Verification items for the finished model (mm, model axes). Coordinates: 2 decimals unless noted, no trailing zeros. Order: outer loops, then holes, each group sorted by start corner. A loop starts at its lowest first (then second) coordinate and runs counter-clockwise, first axis right, second up. Notation, with made-up numbers: (-34.75, 66.5) -> (9.25, 66.5) arc R30 ccw to (9.25, 94.5) -> close; hole circle Ø1 at (4.25, 38.25). An arc over 180 degrees is marked (long way). Answer as CSV lines item,"result".
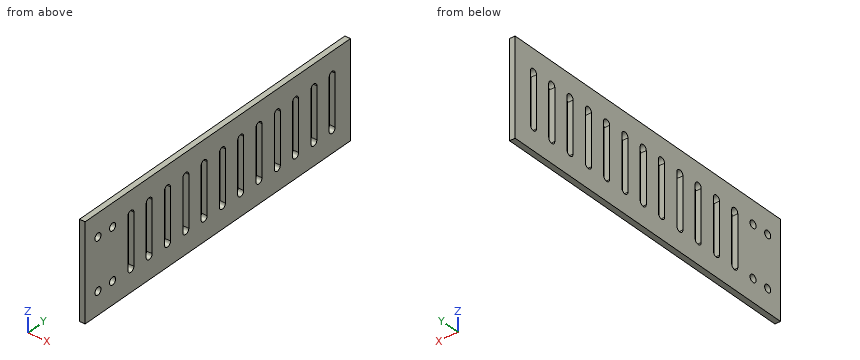
Autodesk Inventor part; units mm, degrees
ref_plane "YZ Plane" through (0, 0, 0) normal (1, 0, 0) x (0, 1, 0)
ref_plane "XZ Plane" through (0, 0, 0) normal (0, 1, 0) x (-1, 0, 0)
ref_plane "XY Plane" through (0, 0, 0) normal (0, 0, 1) x (1, 0, 0)
sketch "Sketch1" plane through (0, 0, 0) normal (1, 0, 0) x (0, 1, 0)
  circle A0 centre (0, -22.5) radius 1.65
  circle A1 centre (-8, 0) radius 1.65
  circle A2 centre (-8, -22.5) radius 1.65
  line L0 (0, 0) -> (-15, 0)
  line L1 (-15, 0) -> (-15, -22.5)
  line L2 (0, -22.5) -> (0, 0)
  line L3 (-15, -22.5) -> (-15, -32.5)
  line L4 (-15, -32.5) -> (0, -32.5)
  line L5 (0, -32.5) -> (0, -22.5)
  line L6 (0, 0) -> (-15, 0)
  line L7 (-15, 0) -> (-15, 10)
  line L8 (-15, 10) -> (0, 10)
  line L9 (0, 10) -> (0, 0)
  line L10 (0, 10) -> (130, 10)
  line L11 (130, 10) -> (130, -32.5)
  line L12 (130, -32.5) -> (0, -32.5)
  line L13 (0, -32.5) -> (0, 10)
  line L14 (10, 0) -> (10, -22.5) construction
  line L15 (8.35, 0) -> (8.35, -22.5)
  line L16 (11.65, -22.5) -> (11.65, 0)
  arc A3 (11.65, 0) -> (8.35, 0) centre (10, 0) ccw
  arc A4 (8.35, -22.5) -> (11.65, -22.5) centre (10, -22.5) ccw
  line L17 (18.35, 0) -> (18.35, -22.5)
  line L18 (20, 0) -> (20, -22.5) construction
  line L19 (21.65, -22.5) -> (21.65, 0)
  arc A5 (21.65, 0) -> (18.35, 0) centre (20, 0) ccw
  arc A6 (18.35, -22.5) -> (21.65, -22.5) centre (20, -22.5) ccw
  line L20 (28.35, 0) -> (28.35, -22.5)
  line L21 (30, 0) -> (30, -22.5) construction
  line L22 (31.65, -22.5) -> (31.65, 0)
  arc A7 (31.65, 0) -> (28.35, 0) centre (30, 0) ccw
  arc A8 (28.35, -22.5) -> (31.65, -22.5) centre (30, -22.5) ccw
  line L23 (38.35, 0) -> (38.35, -22.5)
  line L24 (40, 0) -> (40, -22.5) construction
  line L25 (41.65, -22.5) -> (41.65, 0)
  arc A9 (41.65, 0) -> (38.35, 0) centre (40, 0) ccw
  arc A10 (38.35, -22.5) -> (41.65, -22.5) centre (40, -22.5) ccw
  line L26 (48.35, 0) -> (48.35, -22.5)
  line L27 (50, 0) -> (50, -22.5) construction
  line L28 (51.65, -22.5) -> (51.65, 0)
  arc A11 (51.65, 0) -> (48.35, 0) centre (50, 0) ccw
  arc A12 (48.35, -22.5) -> (51.65, -22.5) centre (50, -22.5) ccw
  line L29 (58.35, 0) -> (58.35, -22.5)
  line L30 (60, 0) -> (60, -22.5) construction
  line L31 (61.65, -22.5) -> (61.65, 0)
  arc A13 (61.65, 0) -> (58.35, 0) centre (60, 0) ccw
  arc A14 (58.35, -22.5) -> (61.65, -22.5) centre (60, -22.5) ccw
  line L32 (68.35, 0) -> (68.35, -22.5)
  line L33 (70, 0) -> (70, -22.5) construction
  line L34 (71.65, -22.5) -> (71.65, 0)
  arc A15 (71.65, 0) -> (68.35, 0) centre (70, 0) ccw
  arc A16 (68.35, -22.5) -> (71.65, -22.5) centre (70, -22.5) ccw
  line L35 (78.35, 0) -> (78.35, -22.5)
  line L36 (80, 0) -> (80, -22.5) construction
  line L37 (81.65, -22.5) -> (81.65, 0)
  arc A17 (81.65, 0) -> (78.35, 0) centre (80, 0) ccw
  arc A18 (78.35, -22.5) -> (81.65, -22.5) centre (80, -22.5) ccw
  line L38 (88.35, 0) -> (88.35, -22.5)
  line L39 (90, 0) -> (90, -22.5) construction
  line L40 (91.65, -22.5) -> (91.65, 0)
  arc A19 (91.65, 0) -> (88.35, 0) centre (90, 0) ccw
  arc A20 (88.35, -22.5) -> (91.65, -22.5) centre (90, -22.5) ccw
  line L41 (98.35, 0) -> (98.35, -22.5)
  line L42 (100, 0) -> (100, -22.5) construction
  line L43 (101.65, -22.5) -> (101.65, 0)
  arc A21 (101.65, 0) -> (98.35, 0) centre (100, 0) ccw
  arc A22 (98.35, -22.5) -> (101.65, -22.5) centre (100, -22.5) ccw
  line L44 (108.35, 0) -> (108.35, -22.5)
  line L45 (110, 0) -> (110, -22.5) construction
  line L46 (111.65, -22.5) -> (111.65, 0)
  arc A23 (111.65, 0) -> (108.35, 0) centre (110, 0) ccw
  arc A24 (108.35, -22.5) -> (111.65, -22.5) centre (110, -22.5) ccw
  line L47 (118.35, 0) -> (118.35, -22.5)
  line L48 (120, 0) -> (120, -22.5) construction
  line L49 (121.65, -22.5) -> (121.65, 0)
  arc A25 (121.65, 0) -> (118.35, 0) centre (120, 0) ccw
  arc A26 (118.35, -22.5) -> (121.65, -22.5) centre (120, -22.5) ccw
  circle A27 centre (0, 0) radius 1.65
  point P0 (10, -11.25)
  point P1 (20, -11.25)
  point P2 (30, -11.25)
  point P3 (40, -11.25)
  point P4 (50, -11.25)
  point P5 (60, -11.25)
  point P6 (70, -11.25)
  point P7 (80, -11.25)
  point P8 (90, -11.25)
  point P9 (100, -11.25)
  point P10 (110, -11.25)
  point P11 (120, -11.25)
  dimension "d1" = 3.3
  dimension "d3" = 3.3
  dimension "d5" = 3.3
  dimension "d6" = 10
  dimension "d7" = 10
  dimension "d9" = 3.3
  dimension "d13" = 10
  dimension "d20" = 15
  dimension "d22" = 7
  dimension "d23" = 7
  dimension "d24" = 8
  dimension "d25" = 3.3
  dimension "d26" = 8
  dimension "d27" = 8
extrude "Extrusion1" add sketch "Sketch1" along normal blind 2.5 contours A0 L2 A27 L9 L10 L11 L12 L5 | A0 L5 L4 L3 L1 L0 A1 A27 L2 | L0 A1 L7 L8 L9 A27
properties part number "Wall Conyevor Depan_3DPrint"
Item 1: Section check A-A, the plane y = 20. Record the boundary of the cut face in (x, z), plus the area to 4 significant figures.
Answer list:
outline,"(0, -32.5) -> (2.5, -32.5) -> (2.5, -24.15) -> (0, -24.15) -> close; (0, 1.65) -> (2.5, 1.65) -> (2.5, 10) -> (0, 10) -> close"
area,"41.75 mm2"
Item 2: Thickness scan on line 1 (Z direction, x = 2.05, y = -8); line 2 (Z direction, x = 0.35, y = 110); line 3 (Z direction, x = 1.9, y = 18.5). Record the ranges inside material, lowest first.
Answer list:
line 1,"-32.5 to -24.15, -20.85 to -1.65, 1.65 to 10"
line 2,"-32.5 to -24.15, 1.65 to 10"
line 3,"-32.5 to -23.19, 0.69 to 10"
Item 3: Section check B-B, the plane z = -8. Count the separate pieces of the cut face and the enclosed holes in it, plus the area to 4 significant figures.
Answer list:
separate pieces,"13"
enclosed holes,"0"
area,"263.5 mm2"
